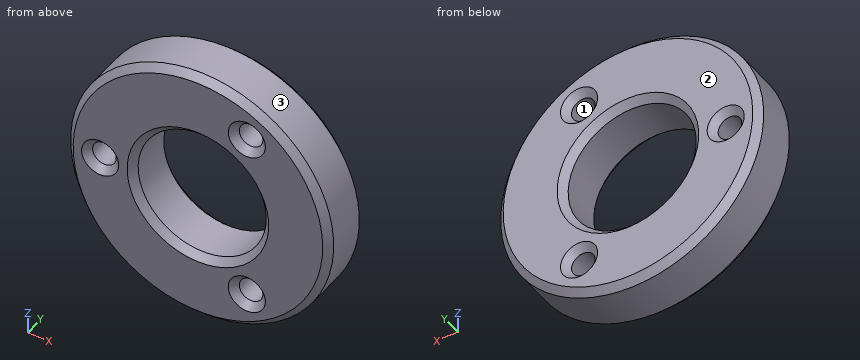
```python
from build123d import *

# Parameters (mm, degrees)
SKETCH1_R           = 19.5
SKETCH1_R_2         = 9.5
SKETCH1_R_3         = 1.75
BOSS_EXTRUDE1_DEPTH = 8
CHAMFER1_SIZE       = 1


with BuildPart() as part:
    # Sketch1 → Boss-Extrude1 (new body)
    with BuildSketch(Plane(origin=(0, 0, 0), x_dir=(1, 0, 0), z_dir=(0, 1, 0))):
        with Locations(Location((0, 0, 0), (0, 0, 270))):
            Circle(SKETCH1_R)
        with Locations(Location((0, 0, 0), (0, 0, 270))):
            Circle(SKETCH1_R_2, mode=Mode.SUBTRACT)
        with Locations(Location((-14.5, 0, 0), (0, 0, 270))):
            Circle(SKETCH1_R_3, mode=Mode.SUBTRACT)
        with Locations(Location((7.25, 12.557368355, 0), (0, 0, 270))):
            Circle(SKETCH1_R_3, mode=Mode.SUBTRACT)
        with Locations(Location((7.25, -12.557368355, 0), (0, 0, 270))):
            Circle(SKETCH1_R_3, mode=Mode.SUBTRACT)
    extrude(amount=BOSS_EXTRUDE1_DEPTH)

    # Chamfer1
    chamfer1_edges = [part.edges().sort_by_distance(p)[0] for p in [
        (7.25, 0, -14.307368355),
        (7.25, 8, -14.307368355),
        (7.25, 0, 10.807368355),
        (7.25, 8, 10.807368355),
        (0, 0, -19.5),
        (0, 8, -19.5),
        (0, 0, -9.5),
        (0, 8, -9.5),
        (-14.5, 0, -1.75),
        (-14.5, 8, -1.75),
    ]]
    chamfer(chamfer1_edges, length=CHAMFER1_SIZE)


solid = part.part
```
The model under review builds one solid part; all positions refer to its coordinate system, in mm. Face numbers are marked on the shaded views. Coordinates: 2 decimals unless noted, no trailing zeros. Write each loop counter-clockwise with the first axis right and the second up, starting at its lowest first coordinate (ties: lowest second). Pieces come first, ordered by that corner, then holes. Notation, with made-up numbers: (7, 50.25) -> (59, 50.25) arc R15 cw to (59, 66.25) -> close; hole circle Ø9 at (73.5, -10). An arc over 180 degrees is marked (long way). One line per item, written item: value. Start each with the question number.
Q1. Add section B-B, the plane y = 5.25. Give the boundary of the cut face in (x, z).
Q2. Add section A-A, the plane z = 0. Give the boundary of the cut face in (x, y).
Q3. Add section D-D, the plane x = 7.25. Count the separate pieces of the cut face and the enclosed holes in it, then the cut area to 3 significant figures.
Q4. The part is to be moulded in two halves that separate along X. For the marked faces 1, 2 and 3, say which applies: +X half, -X half, draft (parallel to the pull), parting line (faces both ways), or undercut.
Q5. Add section C-C, the plane x = 0. Give the boundary of the cut face in (y, z), then the cut area to 3 significant figures.
Q6. Clearance check with flat-ended pins moving along their axes: P1, Ø1.5, axis at x = 11.5, y = 6, coming from the -Z side; P2, Ø3, axis at x = -12.5, y = 4.5, coming from the +Z side; P3, Ø11.5, axis at x = 0, z = 0, coming from the -Y side. State where each tip first meets the part, or that it passes through.
Q7. To check wall thickness, follow probe 1 along X at (y, z) = (3, 0); probe 2 along X at (y, z) = (5.75, -12); probe 3 along X at (y, z) = (5.25, 2.5). State the ranges of each line that lie inside material, in increasing order.
Response:
1. outline: circle Ø39 at (0, 0); hole circle Ø3.5 at (-14.5, 0); hole circle Ø19 at (0, 0); hole circle Ø3.5 at (7.25, -12.56); hole circle Ø3.5 at (7.25, 12.56)
2. outline: (-19.5, 1) -> (-18.5, 0) -> (-17.25, 0) -> (-16.25, 1) -> (-16.25, 7) -> (-17.25, 8) -> (-18.5, 8) -> (-19.5, 7) -> close; (-12.75, 1) -> (-11.75, 0) -> (-10.5, 0) -> (-9.5, 1) -> (-9.5, 7) -> (-10.5, 8) -> (-11.75, 8) -> (-12.75, 7) -> close; (9.5, 1) -> (10.5, 0) -> (18.5, 0) -> (19.5, 1) -> (19.5, 7) -> (18.5, 8) -> (10.5, 8) -> (9.5, 7) -> close
3. separate pieces: 4
3. enclosed holes: 0
3. area: 126 mm²
4. face 1: undercut
4. face 2: draft
4. face 3: parting line
5. outline: (0, -18.5) -> (1, -19.5) -> (7, -19.5) -> (8, -18.5) -> (8, -10.5) -> (7, -9.5) -> (1, -9.5) -> (0, -10.5) -> close; (0, 10.5) -> (1, 9.5) -> (7, 9.5) -> (8, 10.5) -> (8, 18.5) -> (7, 19.5) -> (1, 19.5) -> (0, 18.5) -> close
5. area: 156 mm²
6. P1: z = -16.27
6. P2: z = 16.1
6. P3: through
7. probe 1: -19.5 to -16.25, -12.75 to -9.5, 9.5 to 19.5
7. probe 2: -15.37 to 5.59, 8.91 to 15.37
7. probe 3: -19.34 to -9.17, 9.17 to 19.34
